```python
from build123d import *

# Parameters (mm, degrees)
SKETCH1_W           = 98
SKETCH1_H           = 7
SKETCH1_R           = 1.6
BOSS_EXTRUDE1_DEPTH = 1.2
SKETCH2_W           = 98
SKETCH2_H           = 9.8
SKETCH2_R           = 2.1
BOSS_EXTRUDE2_DEPTH = 1.2


with BuildPart() as part:
    # Sketch1 → Boss-Extrude1 (new body)
    with BuildSketch(Plane.XY):
        Rectangle(SKETCH1_W, SKETCH1_H)
        with Locations((-35, -0.7)):
            Circle(SKETCH1_R, mode=Mode.SUBTRACT)
        with Locations(Location((35, -0.7, 0), (0, 0, 180))):
            Circle(SKETCH1_R, mode=Mode.SUBTRACT)
    extrude(amount=BOSS_EXTRUDE1_DEPTH)

    # Sketch2 → Boss-Extrude2 (add)
    with BuildSketch(Plane(origin=(0, 3.5, 0), x_dir=(1, 0, 0), z_dir=(0, 1, 0))):
        with Locations((0, -6.1)):
            Rectangle(SKETCH2_W, SKETCH2_H)
        with Locations(Location((-43, -6, 0), (0, 0, 270))):
            Circle(SKETCH2_R, mode=Mode.SUBTRACT)
        with Locations(Location((43, -6, 0), (0, 0, 90))):
            Circle(SKETCH2_R, mode=Mode.SUBTRACT)
    extrude(amount=-BOSS_EXTRUDE2_DEPTH)


solid = part.part
```
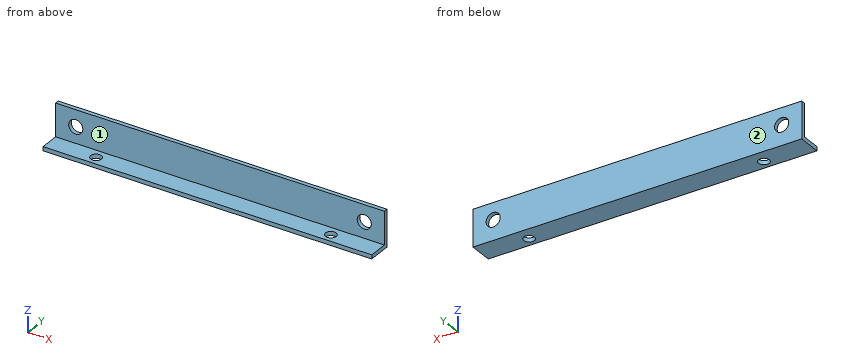
Here's how the part is built. I have some questions about the finished solid (model axes, mm). Face numbers are marked on the shaded views. A direction names the side the tool comes from. Round coordinates to 2 decimals unless told otherwise and drop trailing zeros. Loops run counter-clockwise (first coordinate to the right, second up) from the corner with the lowest first, then second, coordinate; pieces in that order, holes last.
1. Suppose I cut it at A-A, the plane x = -35. Please give me the cut outline in (y, z), and give its area (3 significant figures).
Answers:
outline: (-3.5, 0) - (-2.3, 0) - (-2.3, 1.2) - (-3.5, 1.2) - close; (0.9, 0) - (3.5, 0) - (3.5, 11) - (2.3, 11) - (2.3, 1.2) - (0.9, 1.2) - close
area: 16.3 mm2
2. Suppose I cut it at B-B, the plane z = 5. Please give me the cut outline in (x, y), and give its area (3 significant figures).
Answers:
outline: (-49, 2.3) - (-44.85, 2.3) - (-44.85, 3.5) - (-49, 3.5) - close; (-41.15, 2.3) - (41.15, 2.3) - (41.15, 3.5) - (-41.15, 3.5) - close; (44.85, 2.3) - (49, 2.3) - (49, 3.5) - (44.85, 3.5) - close
area: 109 mm2
3. Will these pins go through, and if not, where does the flat tip stop? pin 1 (1 mm diameter, centred on x = -0.5, z = 5, fed in from -Y); pin 2 (1.7 mm diameter, centred on x = -19.5, y = -1.5, fed in from +Z); pin 3 (2.5 mm diameter, centred on x = 35, y = -0.7, fed in from +Z).
Answers:
pin 1: stops at y = 2.3
pin 2: stops at z = 1.2
pin 3: passes through
4. For the marked faces 1 and 2, which set-ups out of +Z, -Z, +X, -X, +Y, -Y let a thin tool reach every point of the face, with its end or its side?
Answers:
face 1: +Z, +X, -X, -Y
face 2: +Z, -Z, +X, -X, +Y
5. Suppose I cut it at C-C, the plane x = 22. Please give me the cut outline in (y, z).
Answers:
outline: (-3.5, 0) - (3.5, 0) - (3.5, 11) - (2.3, 11) - (2.3, 1.2) - (-3.5, 1.2) - close
6. Suppose I cut it at D-D, the plane z = 10. Please give me the cut outline in (x, y).
Answers:
outline: (-49, 2.3) - (49, 2.3) - (49, 3.5) - (-49, 3.5) - close
7. If I drill on probe 1 along X at (y, z) = (2.75, 6); probe 2 along Y at (x, z) = (35, 0.6); probe 3 along Z at (x, y) = (43, 2.95), over which ranges is the centre line in solid material (lowest first)?
Answers:
probe 1: x = -49 to -45.1, -40.9 to 40.9, 45.1 to 49
probe 2: y = -3.5 to -2.3, 0.9 to 3.5
probe 3: z = 0 to 3.9, 8.1 to 11
